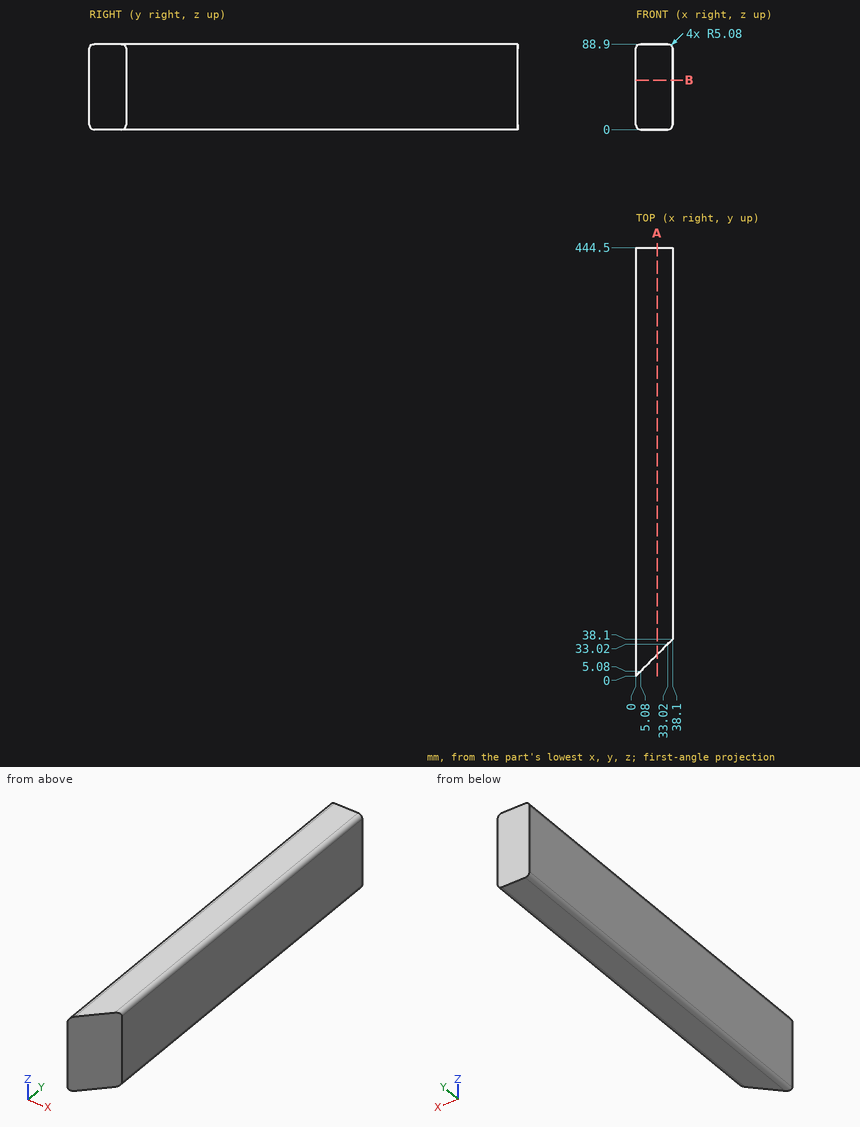
Geometry check sheet. Reference: drawing and pictorial views, mm from the part's lowest x, y, z. Give positions to 0.01 mm unless a question says otherwise; leave off trailing zeros. Loops run counter-clockwise (first coordinate to the right, second up) from the corner with the lowest first, then second, coordinate; pieces in that order, holes last. Notation, with made-up numbers: M -13.75,-26.75 L -5.75,-26.75 A22 cw -5.75,-1.75 Z; hole C 18,52.5 d10. An arc over 180 degrees is marked long. One line per question, with ' | ' between items.
Item 1: Thickness scan on line 1 (Y direction, x = 2.5, z = 4.5); line 2 (Y direction, x = 5, z = 35); line 3 (Z direction, x = 2.5, y = 335.5). Record the ranges inside material, lowest first. Write a range as [from, to].
Completed:
line 1: y = [2.5, 444.5] | line 2: y = [5, 444.5] | line 3: z = [0.7, 88.2]
Item 2: Section check A-A, the plane x = 22. Record the cut outline in (y, z), plus the area to 3 significant figures.
Completed:
outline: M 22,0 L 444.5,0 L 444.5,88.9 L 22,88.9 Z | area: 37,600 mm^2
Item 3: Depth check by flat-ended pin: P1, Ø8, axis at x = 25.5, y = 364, coming from the -Z side; P2, Ø1.5, axis at x = 16.5, z = 41.5, coming from the -Y side. Enter the tip coordinate at first touch or a pass-through.
Completed:
P1: stops at z = 0 | P2: stops at y = 15.75
Item 4: Section check B-B, the plane z = 51.5. Record the cut outline in (x, y).
Completed:
outline: M 0,0 L 38.1,38.1 L 38.1,444.5 L 0,444.5 Z
